For this review, take the finished solid that the model builds, in its own axes (mm). Face numbers are marked on the shaded views. Give positions to 0.01 mm unless a question says otherwise; leave off trailing zeros. Write each loop counter-clockwise with the first axis right and the second up, starting at its lowest first coordinate (ties: lowest second). Pieces come first, ordered by that corner, then holes. Notation, with made-up numbers: (-29.5, -34.75) -> (-4.5, -34.75) arc R24 cw to (-4.5, -1.75) -> close; hole circle Ø10 at (3, 17.5). An arc over 180 degrees is marked (long way). Return JSON: item names as keys, results as strings.
from build123d import *

# Parameters (mm, degrees)
BASE_FLANGE1_DEPTH = 736.092
FILLET1_R          = 2.54
SKETCH3_R          = 2.4765
CUT_EXTRUDE1_DEPTH = 854.182865261
SKETCH4_R          = 2.4765
CUT_EXTRUDE2_DEPTH = 1.2192


# Sheet-metal steps are written as plain solids
with BuildPart() as part:
    # Sketch1 → Base-Flange1 (new body)
    with BuildSketch(Plane.XY):
        with BuildLine():
            Line((-214.3252, -15.875), (-214.3252, -1.27))
            ThreePointArc((-214.3252, -1.27), (-213.953225612, -0.371974388), (-213.0552, 0))
            Line((-213.0552, 0), (213.0552, 0))
            ThreePointArc((213.0552, 0), (213.953225612, -0.371974388), (214.3252, -1.27))
            Line((214.3252, -1.27), (214.3252, -15.875))
            Line((214.3252, -15.875), (215.5444, -15.875))
            Line((215.5444, -15.875), (215.5444, -1.27))
            ThreePointArc((215.5444, -1.27), (214.8153302, 0.4901302), (213.0552, 1.2192))
            Line((213.0552, 1.2192), (-213.0552, 1.2192))
            ThreePointArc((-213.0552, 1.2192), (-214.8153302, 0.4901302), (-215.5444, -1.27))
            Line((-215.5444, -1.27), (-215.5444, -15.875))
            Line((-215.5444, -15.875), (-214.3252, -15.875))
        make_face()
    extrude(amount=BASE_FLANGE1_DEPTH)

    # Fillet1
    fillet1_edges = [part.edges().sort_by_distance(p)[0] for p in [
        (-214.9348, -15.875, 0),
        (214.9348, -15.875, 0),
        (214.9348, -15.875, 736.092),
        (-214.9348, -15.875, 736.092),
    ]]
    fillet(fillet1_edges, radius=FILLET1_R)

    # Sketch3 → Cut-Extrude1 (cut, through all)
    with BuildSketch(Plane(origin=(215.5444, 0, 0), x_dir=(0, 0, -1), z_dir=(1, 0, 0))):
        with Locations((-368.3, -8.3058)):
            Circle(SKETCH3_R)
        with Locations((-723.9, -8.3058)):
            Circle(SKETCH3_R)
        with Locations((-12.7, -8.3058)):
            Circle(SKETCH3_R)
    extrude(amount=-CUT_EXTRUDE1_DEPTH, mode=Mode.SUBTRACT)

    # Sketch4 → Cut-Extrude2 (cut)
    with BuildSketch(Plane(origin=(0, 1.2192, 0), x_dir=(1, 0, 0), z_dir=(0, 1, 0))):
        with Locations(Location((-190.5, -12.7, 0), (0, 0, 180))):
            Circle(SKETCH4_R)
        with Locations(Location((0, -12.7, 0), (0, 0, 180))):
            Circle(SKETCH4_R)
        with Locations(Location((190.5, -12.7, 0), (0, 0, 180))):
            Circle(SKETCH4_R)
    extrude(amount=-CUT_EXTRUDE2_DEPTH, mode=Mode.SUBTRACT)


solid = part.part
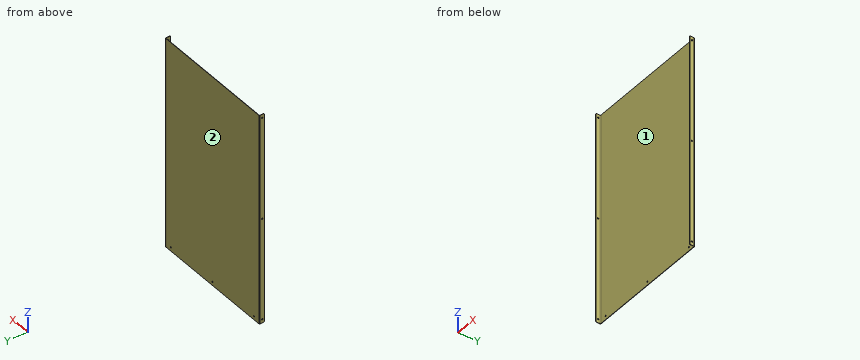
1. Add section B-B, the plane x = -107.5. State the section outline as (y, z) points.
Results found:
{"outline": "(0, 0) -> (1.22, 0) -> (1.22, 736.09) -> (0, 736.09) -> close"}
2. The part is to be moulded in two halves that separate along X. For the marked faces 1 and 2, say which applies: +X half, -X half, draft (parallel to the pull), parting line (faces both ways), or undercut.
Results found:
{"face 1": "undercut", "face 2": "draft"}
3. Add section A-A, the plane z = 280. State the section outline as (x, y) points (3 decimals), plus the area to 3 significant figures.
Results found:
{"outline": "(-215.544, -15.875) -> (-214.325, -15.875) -> (-214.325, -1.27) arc R1.27 cw to (-213.055, 0) -> (213.055, 0) arc R1.27 cw to (214.325, -1.27) -> (214.325, -15.875) -> (215.544, -15.875) -> (215.544, -1.27) arc R2.489 ccw to (213.055, 1.219) -> (-213.055, 1.219) arc R2.489 ccw to (-215.544, -1.27) -> close", "area": "562 mm²"}
4. To check wall thickness, follow probe 1 along X at (y, z) = (-13.5, 539); probe 2 along Z at (x, y) = (0, 0.4); probe 3 along Y at (x, z) = (215.1, 12.7) (3 decimals). State the ranges of each line that lie inside material, in increasing order.
Results found:
{"probe 1": "x = -215.54 to -214.33, 214.33 to 215.54", "probe 2": "z = 0 to 10.22, 15.18 to 736.09", "probe 3": "y = -15.875 to -10.782, -5.829 to 0.149"}
5. For pin 1 (3 mm diameter, centred on y = -8.31, z = 12.7, fed in from -X); pin 2 (5.5 mm diameter, centred on y = -8.31, z = 12.7, fed in from +X); pin 3 (5 mm diameter, centred on x = -134.5, z = 259, fed in from -Y), all flat-tipped, find the tip position at first contact; note any pin that passes through.
Results found:
{"pin 1": "passes through", "pin 2": "stops at x = 215.54", "pin 3": "stops at y = 0"}
